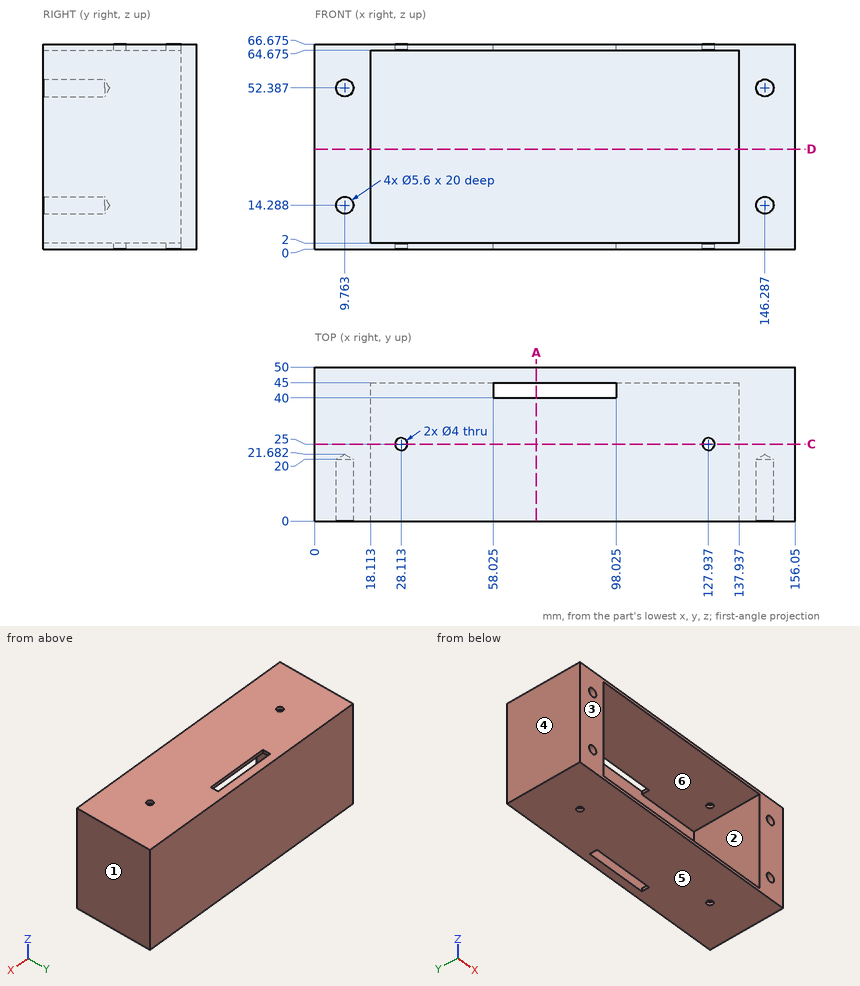
Geometry check sheet. Reference: drawing and pictorial views, mm from the part's lowest x, y, z. A direction names the side the tool comes from. Give positions to 0.01 mm unless a question says otherwise; leave off trailing zeros. Loops run counter-clockwise (first coordinate to the right, second up) from the corner with the lowest first, then second, coordinate; pieces in that order, holes last. Notation, with made-up numbers: M 64.5,-34 L 82.5,-34 A26 cw 82.5,-1 Z; hole C 12,71 d6. An arc over 180 degrees is marked long. Use a Markdown table: item, result. Add a question column.
Q1. Scan lines: line 1 along X through (y, z) = (25, 0.9); line 2 along Z through (x, y) = (81, 26.5) (1 decimal); line 3 along X through (y, z) = (41, 61.5). Record each from-to range of solid material in increasing order. Write a range as [from, to].
Q2. Sectioned sample at D-D, the plane z = 32.5. Record the cut outline in (x, y), then the cut area to 3 significant figures.
Q3. Sectioned sample at C-C, the plane y = 25. Give the number of separate pieces and of enclosed holes in the cut face, then the cut area to 3 significant figures.
Q4. Go/stop test with flat-tipped pins: pin 1 (20 mm diameter, centred on x = 59.5, z = 22, fed in from -Y); pin 2 (3.5 mm diameter, centred on x = 9.763, z = 52.387, fed in from -Y). Record where each tip stops, or that it passes through.
Q5. Sectioned sample at A-A, the plane x = 72. Record the cut outline in (y, z) (1 decimal).
Q6. Mould release check, pull along X, two halves, no side actions. Record for the marked faces 1, 2, 3 and 4: pulls with the +X half, pulls with the -X half, needs draft (parallel to the pull), parting line crosses it, or undercut.
Q7. Tool access check on the marked faces 5 and 6. Record the directions out of +Z, -Z, +X, -X, +Y, -Y that give a thin tool (end or side, any length) a straight path to the whole face; none if there is none.
Verdict:
| question | item | result |
|---|---|---|
| 1 | line 1 | [0, 26.11], [30.11, 125.94], [129.94, 156.05] |
| 1 | line 2 | [0, 2], [64.7, 66.7] |
| 1 | line 3 | [0, 18.11], [137.94, 156.05] |
| 2 | outline | M 0,0 L 18.11,0 L 18.11,45 L 137.94,45 L 137.94,0 L 156.05,0 L 156.05,50 L 0,50 Z |
| 2 | area | 2,410 mm^2 |
| 3 | separate pieces | 4 |
| 3 | enclosed holes | 0 |
| 3 | area | 2,860 mm^2 |
| 4 | pin 1 | y = 45 |
| 4 | pin 2 | y = 20.63 |
| 5 | outline | M 0,0 L 40,0 L 40,2 L 0,2 Z; M 0,64.7 L 40,64.7 L 40,66.7 L 0,66.7 Z; M 45,0 L 50,0 L 50,66.7 L 45,66.7 Z |
| 6 | face 1 | pulls with the +X half |
| 6 | face 2 | undercut |
| 6 | face 3 | needs draft |
| 6 | face 4 | pulls with the -X half |
| 7 | face 5 | -Z, +X, -X, +Y, -Y |
| 7 | face 6 | -Y |
